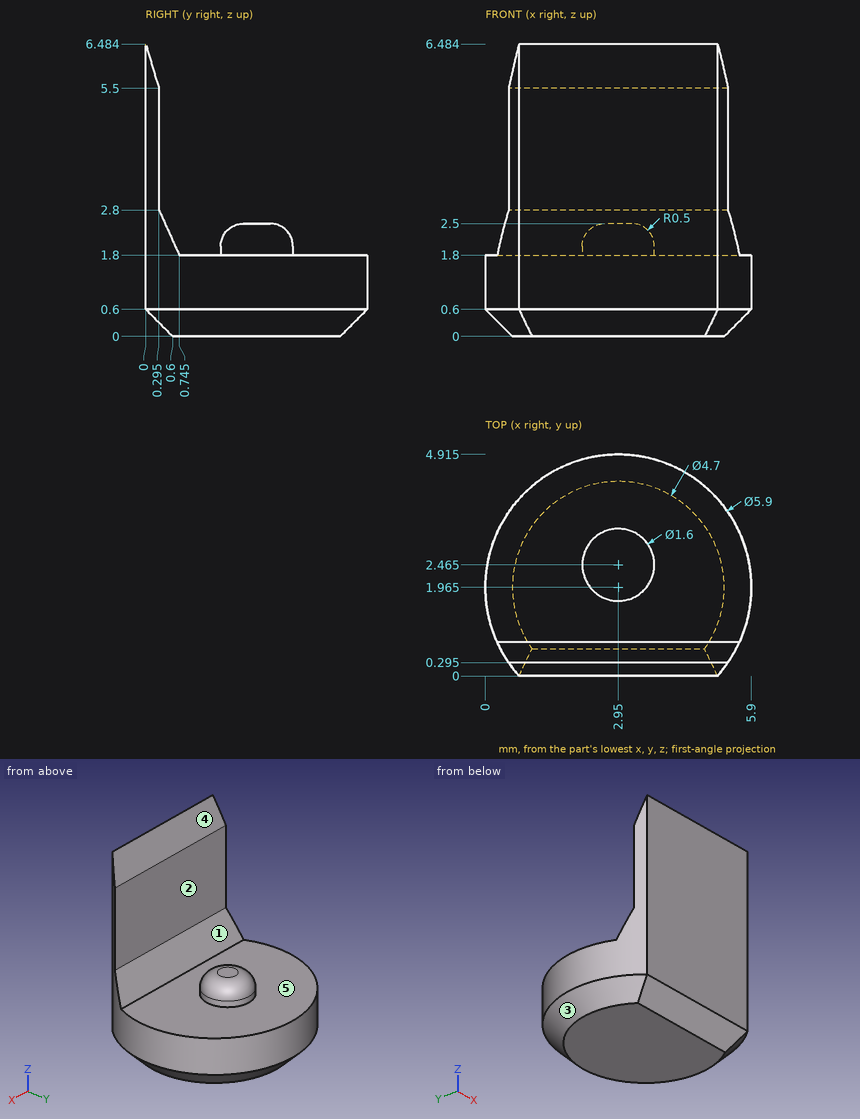
Answer from the drawing. Dimensions are ordinates in mm from the lowest x, y and z of the part. A direction names the side the tool comes from. Coordinates: 2 decimals unless noted, no trailing zeros. Put each result on its own line as item: value. Start each with the question number.
1. For a pull along Y with two mould halves and no side action, classify the marked faces 1, 2 and 3 as pulls with the +Y half, pulls with the -Y half, needs draft (parallel to the pull), parting line crosses it, or undercut.
2. Which of the six approach directions +Z, -Z, +X, -X, +Y, -Y give full straight-line access (tool end or side, diameter ignored) to the marked faces 4 and 5?
3. Flat-ended cylindrical pins translate along their axes: P1, Ø1.5, axis at y = 2, z = 3, coming from the -X side; P2, Ø1.4, axis at x = 4, z = 4, coming from the +Y side (1 decimal); P3, Ø2, axis at x = 4.5, y = 2, coming from the +Z side (1 decimal). Find the tip coordinate at first contact, or state that the pin passes through.
4. Consider line 1 (Z direction, x = 0.8, y = 3.5); line 2 (Y direction, x = 3.4, z = 3) (1 decimal); line 3 (Z direction, x = 4.05, y = 0.95). Determine where each line is inside the solid, lowest interval first. Write a range as from..to.
Resolved:
1. face 1: undercut
1. face 2: pulls with the +Y half
1. face 3: parting line crosses it
2. face 4: +Z, +X, -X, +Y
2. face 5: +Z
3. P1: stops at x = 2.28
3. P2: stops at y = 0.3
3. P3: stops at z = 2.4
4. line 1: z = 0.29..1.8
4. line 2: y = 0..0.3
4. line 3: z = 0..1.8
